```python
from build123d import *

# Parameters (mm, degrees)
F0_W     = 25
F0_H     = 18.8
F0_R     = 1.8
F1_DEPTH = 4
F0_H_2   = 4
F2_DEPTH = 40
F3_W     = 25
F3_H     = 4
F4_DEPTH = 25
F5_R     = 9.25
F6_DEPTH = 4
F7_R     = 12.49999
F8_SIZE  = 6


# Not quite as in the source:
# - a fillet or chamfer is up to 0.001 mm smaller than in the source, because OpenCascade refuses the exact size


with BuildPart() as f1:
    # F0 (on Top) → F1 (new body)
    with BuildSketch(Plane.XY):
        with Locations((0, -9.4)):
            Rectangle(F0_W, F0_H)
        with Locations((0, -3.8)):
            Circle(F0_R, mode=Mode.SUBTRACT)
    extrude(amount=F1_DEPTH)

    # F0 (on Top) → F2 (join)
    with BuildSketch(Plane.XY):
        with Locations((0, -20.8)):
            Rectangle(F0_W, F0_H_2)
    extrude(amount=F2_DEPTH)

    # F3 (on face) → F4 (join)
    with BuildSketch(Plane.XZ.offset(22.8)):
        with Locations((0, 38)):
            Rectangle(F3_W, F3_H)
    extrude(amount=F4_DEPTH)

    # F5 (on face) → F6 (cut, through all)
    with BuildSketch(Plane(origin=(0, 0, 36), x_dir=(1, 0, 0), z_dir=(0, 0, -1))):
        with Locations((0, 35.3)):
            Circle(F5_R)
    extrude(amount=-F6_DEPTH, mode=Mode.SUBTRACT)

    # F7 (radius 12.5 in the source; OpenCascade refuses exactly that, so slightly less here)
    f7_edges = [f1.edges().sort_by_distance(p)[0] for p in [
        (12.5, -47.8, 38),
        (-12.5, -47.8, 38),
    ]]
    fillet(f7_edges, radius=F7_R)

    # F8
    f8_edges = [f1.edges().sort_by_distance(p)[0] for p in [
        (12.5, 0, 2),
        (-12.5, 0, 2),
    ]]
    chamfer(f8_edges, length=F8_SIZE)


solid = f1.part
```
For this review, take the finished solid that the model builds, in its own axes (mm). A direction names the side the tool comes from. Coordinates: 2 decimals unless noted, no trailing zeros. Loops run counter-clockwise (first coordinate to the right, second up) from the corner with the lowest first, then second, coordinate; pieces in that order, holes last. Notation, with made-up numbers: (40, -35) -> (50, -35) arc R6 ccw to (50, -31) -> close; hole circle Ø4 at (27, 10). An arc over 180 degrees is marked (long way). Return JSON: item names as keys, results as strings. Group by question number.
(1) Consider section A-A, the plane y = -3.8. Give the boundary of the cut face in (x, z), plus the area to 3 significant figures.
(2) To check wall thickness, follow L1, parallel to X at y = -35.3, z = 38.9; L2, parallel to Y at x = 0, z = 2.55; L3, parallel to Y at x = 0, z = 38.95. State the ranges of each line that lie inside material, in increasing order.
(3) Consider section D-D, the plane x = 8.5. Give the boundary of the cut face in (y, z), plus the area to 3 significant figures.
(4) Consider section C-C, the plane z = 25. Give the boundary of the cut face in (x, y).
(5) Consider section B-B, the plane x = 5.25. Give the boundary of the cut face in (y, z), plus the area to 3 significant figures.
(6) For pin 1 Ø12.5 at (x, z) = (3.5, 13) entering from -Y; pin 2 Ø12.5 at (x, y) = (-4, -31) entering from -Z; pin 3 Ø4 at (x, y) = (0, -3.8) entering from +Z, all flat-tipped, find the tip position at first contact; note any pin that passes through.
(7) Mouldability with a two-part tool opening along Y and no side actions: class faces 4 (the cylindrical face through (8.741, -44.235, 38.028)), 5 (the flat face through (-9.5, -3, 2)), 6 (the cylindrical face through (-0.39, -5.557, 1.972)), 7 (the cylindrical face through (-2.01, -26.27, 37.97)) as pulls with the +Y half, pulls with the -Y half, needs draft (parallel to the pull), parting line crosses it, or undercut.
(8) Tool access review of faces 1 (the flat face through (5, -27, 36)), 2 (the flat face through (12.5, -21, 20)), 3 (the flat face through (0, -9, 4)): name each direction out of +Z, -Z, +X, -X, +Y, -Y from which nothing blocks a thin tool from reaching the whole face with its end or side.
Results below:
{
 "1": {"outline": "(-10.3, 0) -> (-1.8, 0) -> (-1.8, 4) -> (-10.3, 4) -> close; (1.8, 0) -> (10.3, 0) -> (10.3, 4) -> (1.8, 4) -> close", "area": "68.0 mm2"},
 "2": {"L1": "x = -12.5 to -9.25, 9.25 to 12.5", "L2": "y = -22.8 to -5.6, -2 to 0", "L3": "y = -47.8 to -44.55, -26.05 to -18.8"},
 "3": {"outline": "(-44.47, 36) -> (-38.95, 36) -> (-38.95, 40) -> (-44.47, 40) -> close; (-31.65, 36) -> (-22.8, 36) -> (-22.8, 0) -> (-2, 0) -> (-2, 4) -> (-18.8, 4) -> (-18.8, 40) -> (-31.65, 40) -> close", "area": "285 mm2"},
 "4": {"outline": "(-12.5, -22.8) -> (12.5, -22.8) -> (12.5, -18.8) -> (-12.5, -18.8) -> close"},
 "5": {"outline": "(-46.64, 36) -> (-42.92, 36) -> (-42.92, 40) -> (-46.64, 40) -> close; (-27.68, 36) -> (-22.8, 36) -> (-22.8, 0) -> (0, 0) -> (0, 4) -> (-18.8, 4) -> (-18.8, 40) -> (-27.68, 40) -> close", "area": "270 mm2"},
 "6": {"pin 1": "stops at y = -22.8", "pin 2": "stops at z = 36", "pin 3": "stops at z = 4"},
 "7": {"face 4": "pulls with the -Y half", "face 5": "pulls with the +Y half", "face 6": "undercut", "face 7": "undercut"},
 "8": {"face 1": "-Z, +X, -X, -Y", "face 2": "+Z, -Z, +X, +Y, -Y", "face 3": "+Z, +X, -X, +Y"}
}
